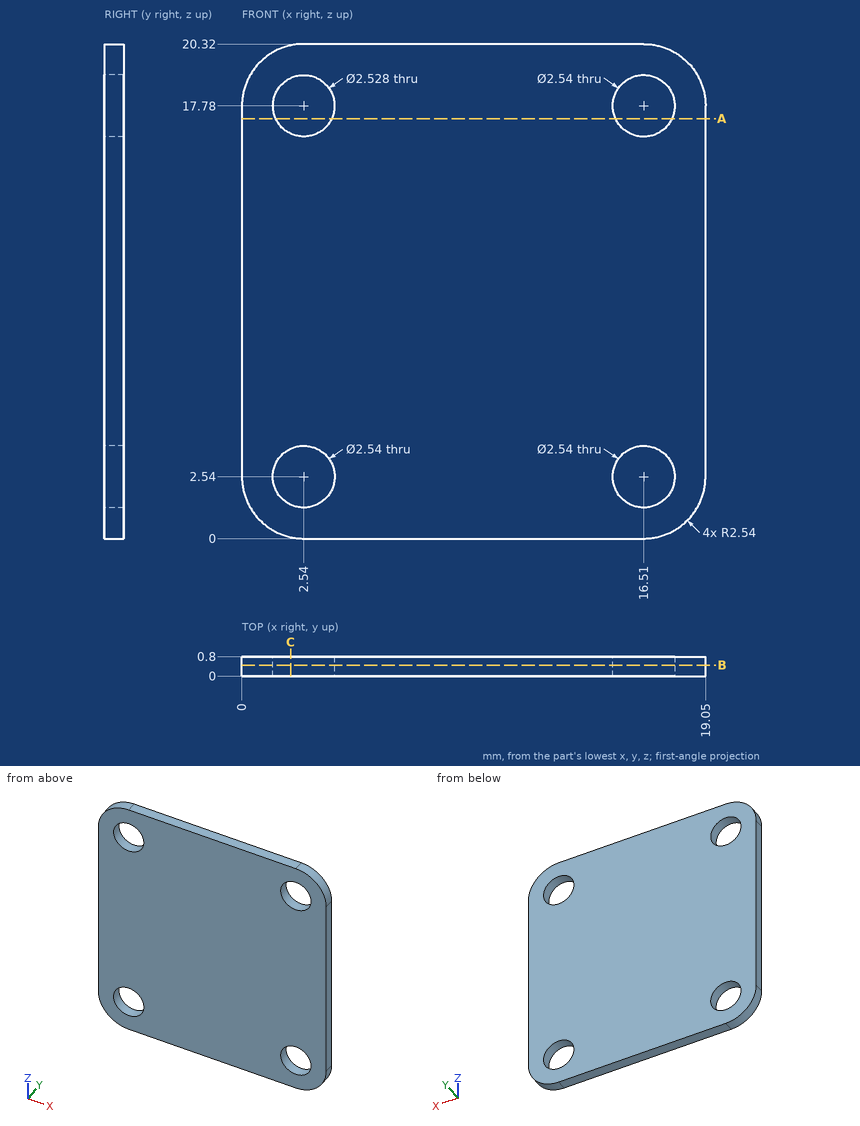
Job drawing, mm, ordinate dimensions from the low corner. One solid piece. Give positions to 0.01 mm unless a question says otherwise; leave off trailing zeros. Write each loop counter-clockwise with the first axis right and the second up, starting at its lowest first coordinate (ties: lowest second). Pieces come first, ordered by that corner, then holes. Notation, with made-up numbers: M 0.25,83.5 L 14.25,83.5 A18 ccw 14.25,90.5 Z; hole C 21.25,42.25 d5. An arc over 180 degrees is marked long. Put each result on its own line as item: value. Start each with the question number.
(1) Band-saw the part on B-B, the plane y = 0.45. Write the cut outline in (x, z), and give its area (3 significant figures).
(2) Band-saw the part on C-C, the plane x = 2. Write the cut outline in (y, z), and give its area (3 significant figures).
(3) Probe L1, parallel to Z at x = 16.51, y = 0.45; L2, parallel to Z at x = 3.25, y = 0.3 (1 decimal); L3, parallel to X at y = 0.15, z = 17.5. List the from-to ranges inside material, lowest first.
(4) Band-saw the part on A-A, the plane z = 17.25. Write the cut outline in (x, y).
Response values:
1. outline: M 0,2.54 A2.54 ccw 2.54,0 L 16.51,0 A2.54 ccw 19.05,2.54 L 19.05,17.78 A2.54 ccw 16.51,20.32 L 2.54,20.32 A2.54 ccw 0,17.78 Z; hole C 2.54,2.54 d2.54; hole C 2.54,17.78 d2.53; hole C 16.51,2.54 d2.54; hole C 16.51,17.78 d2.54
1. area: 361 mm2
2. outline: M 0,0.06 L 0.8,0.06 L 0.8,1.39 L 0,1.39 Z; M 0,3.69 L 0.8,3.69 L 0.8,16.64 L 0,16.64 Z; M 0,18.92 L 0.8,18.92 L 0.8,20.26 L 0,20.26 Z
2. area: 12.5 mm2
3. L1: z = 0 to 1.27, 3.81 to 16.51, 19.05 to 20.32
3. L2: z = 0 to 1.5, 3.6 to 16.7, 18.8 to 20.3
3. L3: x = 0 to 1.31, 3.77 to 15.27, 17.75 to 19.05
4. outline: M 0,0 L 1.39,0 L 1.39,0.8 L 0,0.8 Z; M 3.69,0 L 15.36,0 L 15.36,0.8 L 3.69,0.8 Z; M 17.66,0 L 19.05,0 L 19.05,0.8 L 17.66,0.8 Z
